Work out the finished part from the listing and answer in its coordinate system (mm). A direction names the side the tool comes from. Coordinates: 2 decimals unless noted, no trailing zeros. Write each loop counter-clockwise with the first axis right and the second up, starting at its lowest first coordinate (ties: lowest second). Pieces come first, ordered by that corner, then holes. Notation, with made-up numbers: (-19.75, -18) - (25.25, -18) arc R15 cw to (25.25, -13) - close; hole circle Ø1 at (-22.75, -30). An arc over 180 degrees is marked (long way). Use one line per item in the form item = value. Start each with the question number.
Item 1: Consider probe 1 along Y at (x, z) = (12.5, 6.5); probe 2 along Y at (x, z) = (12.5, 8.5); probe 3 along X at (y, z) = (-7.25, 14.25). Determine where each line is inside the solid, lowest interval first.
Item 2: A cutting plane is placed at B-B (x = -12.5). Write down the section's boundary in (y, z), then the cut area to 3 significant figures.
Item 3: A cutting plane is placed at D-D (x = -6.5). Write down the section's boundary in (y, z).
Item 4: A cutting plane is placed at A-A (z = 12.5). Write down the section's boundary in (x, y), then the cut area to 3 significant figures.
Item 5: Determine the mould class of faces 3 (the flat face through (10, 4, 13)), 4 (the flat face through (0, -15, 1)), 5 (the cylindrical face through (-22.04, -3, 9.4)), 6 (the flat face through (0, 15, 1)) for opening direction Y: released by +Y, released by -Y, zero draft, split by the parting line, or undercut.
Item 6: A cutting plane is placed at C-C (y = -9.5). Write down the section's boundary in (x, z), then the cut area to 3 significant figures.
Item 7: Given pin 1 (3 mm diameter, centred on x = -10.5, y = 2, fed in from +Z); pin 2 (1 mm diameter, centred on y = -6, z = 10.5, fed in from +X); pin 3 (4 mm diameter, centred on y = -10, z = 4.5, fed in from -X), each flat-ended and moving along its own axis, determine where each tip first touches the part or whether it passes through.
Item 8: For faces 1 (the flat face through (21, -4, 17)), 2 (the flat face through (-14, 5, 8)), determine the directions among +Z, -Z, +X, -X, +Y, -Y from which every point of the face is accessible in a straight line to the end or side of a thin tool.
from build123d import *

# Parameters (mm, degrees)
SKETCH_1_W      = 50
SKETCH_1_H      = 30
EXTRUDE_1_DEPTH = 2
SKETCH_2_R      = 10
SKETCH_2_R_2    = 9
EXTRUDE_2_DEPTH = 15
SKETCH_3_R      = 7.5
EXTRUDE_3_DEPTH = 6
SKETCH_4_R      = 5
EXTRUDE_4_DEPTH = 5


with BuildPart() as part:
    # 草图1 → 凸台-拉伸1 (new body)
    with BuildSketch(Plane.XY):
        Rectangle(SKETCH_1_W, SKETCH_1_H)
    extrude(amount=EXTRUDE_1_DEPTH)

    # 草图2 → 凸台-拉伸2 (add)
    # profile 1 of 2: a face of its own
    with BuildSketch(Plane.XY.offset(2)):
        with Locations(Location((12.5, 0, 0), (0, 0, 180))):
            Circle(SKETCH_2_R)
        with Locations((12.5, 0)):
            Circle(SKETCH_2_R_2, mode=Mode.SUBTRACT)
    # profile 2 of 2: a face of its own
    with BuildSketch(Plane.XY.offset(2)):
        with Locations(Location((-12.5, 0, 0), (0, 0, 180))):
            Circle(SKETCH_2_R)
        with Locations(Location((-12.5, 0, 0), (0, 0, 180))):
            Circle(SKETCH_2_R_2, mode=Mode.SUBTRACT)
    extrude(amount=EXTRUDE_2_DEPTH)

    # 草图3 → 凸台-拉伸3 (add)
    with BuildSketch(Plane.XY.offset(2)):
        with Locations(Location((12.5, 0, 0), (0, 0, 180))):
            Circle(SKETCH_3_R)
        with Locations(Location((-12.5, 0, 0), (0, 0, 180))):
            Circle(SKETCH_3_R)
    extrude(amount=EXTRUDE_3_DEPTH)

    # 草图4 → 凸台-拉伸4 (add)
    with BuildSketch(Plane.XY.offset(8)):
        with Locations((-12.5, 0)):
            Circle(SKETCH_4_R)
        with Locations((12.5, 0)):
            Circle(SKETCH_4_R)
    extrude(amount=EXTRUDE_4_DEPTH)

    # 草图5 → 切除-旋转1 (revolve, cut)
    with BuildSketch(Plane(origin=(0, 0, 0), x_dir=(1, 0, 0), z_dir=(0, 1, 0))):
        Polygon((12.5, -13), (17, -13), (13, -11), (12.5, -11), align=None)
    cut_revolve_1 = revolve(axis=Axis((12.5, 0, 14.465329718), (0, 0, -1)), mode=Mode.SUBTRACT)

    # 镜向1: 切除-旋转1 across plane
    add(cut_revolve_1.mirror(Plane(origin=(0, 0, 0), x_dir=(0, 0, 1), z_dir=(1, 0, 0))), mode=Mode.SUBTRACT)


solid = part.part
Answer:
q1.probe_1 = -10 to -9, -7.5 to 7.5, 9 to 10
q1.probe_2 = -10 to -9, -5 to 5, 9 to 10
q1.probe_3 = -19.39 to -17.83, -7.17 to -5.61, 5.61 to 7.17, 17.83 to 19.39
q2.outline = (-15, 0) - (15, 0) - (15, 2) - (10, 2) - (10, 17) - (9, 17) - (9, 2) - (7.5, 2) - (7.5, 8) - (5, 8) - (5, 13) - (4.5, 13) - (0.5, 11) - (-0.5, 11) - (-4.5, 13) - (-5, 13) - (-5, 8) - (-7.5, 8) - (-7.5, 2) - (-9, 2) - (-9, 17) - (-10, 17) - (-10, 2) - (-15, 2) - close
q2.area = 220 mm²
q3.outline = (-15, 0) - (15, 0) - (15, 2) - (8, 2) - (8, 17) - (6.71, 17) - (6.71, 2) - (4.5, 2) - (4.5, 8) - (-4.5, 8) - (-4.5, 2) - (-6.71, 2) - (-6.71, 17) - (-8, 17) - (-8, 2) - (-15, 2) - close
q4.outline = circle Ø20 at (-12.5, 0); circle Ø10 at (-12.5, 0); circle Ø20 at (12.5, 0); circle Ø10 at (12.5, 0); hole circle Ø18 at (-12.5, 0); hole circle Ø7 at (-12.5, 0); hole circle Ø18 at (12.5, 0); hole circle Ø7 at (12.5, 0)
q4.area = 199 mm²
q5.face_3 = undercut
q5.face_4 = released by -Y
q5.face_5 = split by the parting line
q5.face_6 = released by +Y
q6.outline = (-25, 0) - (25, 0) - (25, 2) - (15.62, 2) - (15.62, 17) - (9.38, 17) - (9.38, 2) - (-9.38, 2) - (-9.38, 17) - (-15.62, 17) - (-15.62, 2) - (-25, 2) - close
q6.area = 287 mm²
q7.pin_1 = 12.91
q7.pin_2 = 20.85
q7.pin_3 = -18.5
q8.face_1 = +Z, +X, -X, +Y, -Y
q8.face_2 = +Z
